Source: three-view drawing plus pictorial views. Frame: mm from the lowest corner of the part. A direction names the side the tool comes from. Round coordinates to 2 decimals unless told otherwise and drop trailing zeros. Loops run counter-clockwise (first coordinate to the right, second up) from the corner with the lowest first, then second, coordinate; pieces in that order, holes last. Notation, with made-up numbers: (13.5, 81) -> (40.5, 81) arc R19 cw to (40.5, 94) -> close; hole circle Ø11 at (-21.5, -3). An arc over 180 degrees is marked (long way). Put each result on its own line as item: value. Start each with the question number.
1. Cut plane C-C (y = 15). Return the cut outline in (x, z) (3 decimals).
2. Cut plane D-D (y = 11.5). Return the cut outline in (x, z) (3 decimals).
3. Set-up query: the marked faces 1 and 2. Return all of +Z, -Z, +X, -X, +Y, -Y with unobstructed straight access to the full face (end or side cutting, diameter ignored); none if empty.
4. Contact query for flat-ended pins moving along their axis: pin 1 (1.5 mm diameter, centred on x = 16, y = 3.5, fed in from +Z); pin 2 (1.5 mm diameter, centred on y = 11, z = 30.5, fed in from -X); pin 3 (1.5 mm diameter, centred on y = 11, z = 29, fed in from -X). Output: stop coordinate, or through.
5. Cut plane B-B (x = 20). Return the cut outline in (y, z) (3 decimals).
6. Material intervals for L1, parallel to Z at x = 20, y = 8.25 (3 decimals); L2, parallel to Y at x = 35, z = 27.5, sorted ascending.
7. Draft query along Z for the marked faces 3, 4 and 5. Return one class per face: pulls with the +Z half, pulls with the -Z half, needs draft (parallel to the pull), parting line crosses it, or undercut.
8. Cut plane A-A (z = 20). Return the cut outline in (x, y) (3 decimals), then the cut area to 3 significant figures.
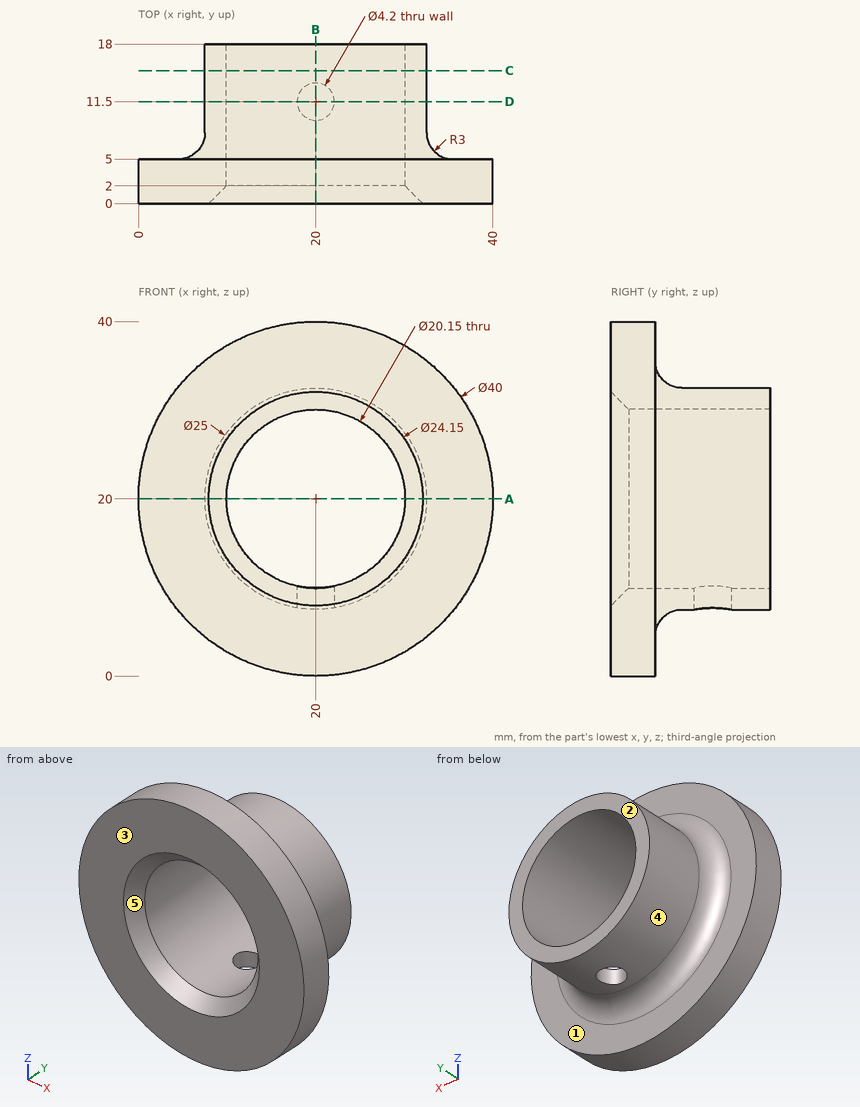
Solution:
1. outline: circle Ø25 at (20, 20); hole circle Ø20.15 at (20, 20)
2. outline: (17.9, 7.678) -> (17.9, 10.146) arc R10.075 cw (long way) to (22.1, 10.146) -> (22.1, 7.678) arc R12.5 ccw (long way) to start
3. face 1: +Y
3. face 2: +Z, -Z, +X, -X, +Y
4. pin 1: stops at z = 39.73
4. pin 2: stops at x = 12.18
4. pin 3: stops at x = 10.61
5. outline: (0, 0) -> (5, 0) -> (5, 4.5) arc R3 cw to (8, 7.5) -> (9.4, 7.5) -> (9.4, 9.925) -> (2, 9.925) -> (0, 7.925) -> close; (0, 32.075) -> (2, 30.075) -> (18, 30.075) -> (18, 32.5) -> (8, 32.5) arc R3 cw to (5, 35.5) -> (5, 40) -> (0, 40) -> close; (13.6, 7.5) -> (18, 7.5) -> (18, 9.925) -> (13.6, 9.925) -> close
6. L1: z = 7.5 to 9.925, 30.075 to 32.5
6. L2: y = 0 to 5
7. face 3: needs draft
7. face 4: parting line crosses it
7. face 5: undercut
8. outline: (0, 0) -> (7.925, 0) -> (9.925, 2) -> (9.925, 18) -> (7.5, 18) -> (7.5, 8) arc R3 cw to (4.5, 5) -> (0, 5) -> close; (30.075, 2) -> (32.075, 0) -> (40, 0) -> (40, 5) -> (35.5, 5) arc R3 cw to (32.5, 8) -> (32.5, 18) -> (30.075, 18) -> close
8. area: 162 mm^2
